For this review, use the dimensioned drawing (mm, ordinates from the lowest corner) and the shaded views. Coordinates: 2 decimals unless noted, no trailing zeros. Loops run counter-clockwise (first coordinate to the right, second up) from the corner with the lowest first, then second, coordinate; pieces in that order, holes last. Notation, with made-up numbers: (58.25, 52.25) - (80.25, 52.25) arc R13 cw to (80.25, 73.25) - close; hole circle Ø8 at (46.25, -36.5). An arc over 180 degrees is marked (long way). Use a Markdown table: item, result. Add a question column.
1) Add section A-A, the plane y = 15. Give the boundary of the cut face in (x, z).
2) Add section B-B, the plane x = 30. Give the boundary of the cut face in (y, z), and give its area (3 significant figures).
3) Clearance check with flat-ended pins moving along their axes: pin 1 (1.5 mm diameter, centred on y = 25.5, z = 3, fed in from +X); pin 2 (4 mm diameter, centred on x = 31, y = 15.5, fed in from -Z); pin 3 (1 mm diameter, centred on x = 22.5, z = 7.5, fed in from +Y); pin 4 (5 mm diameter, centred on x = 29.5, z = 3, fed in from +Y). State where each tip first meets the part, or that it passes through.
4) The part is to be moulded in two halves that separate along Y. For the marked faces 1, 2 and 3, say which applies: pulls with the +Y half, pulls with the -Y half, needs draft (parallel to the pull), parting line crosses it, or undercut.
5) To check wall thickness, follow L1, parallel to Z at x = 57, y = 24; L2, parallel to Y at x = 30, z = 7; L3, parallel to X at y = 3.75, z = 12.25 (1 decimal). State the ranges of each line that lie inside material, in increasing order. Write a range as [from, to].
6) Add section D-D, the plane z = 11.25. Give the boundary of the cut face in (x, y), and give its area (3 significant figures).
7) Add section C-C, the plane z = 4. Give the boundary of the cut face in (x, y).
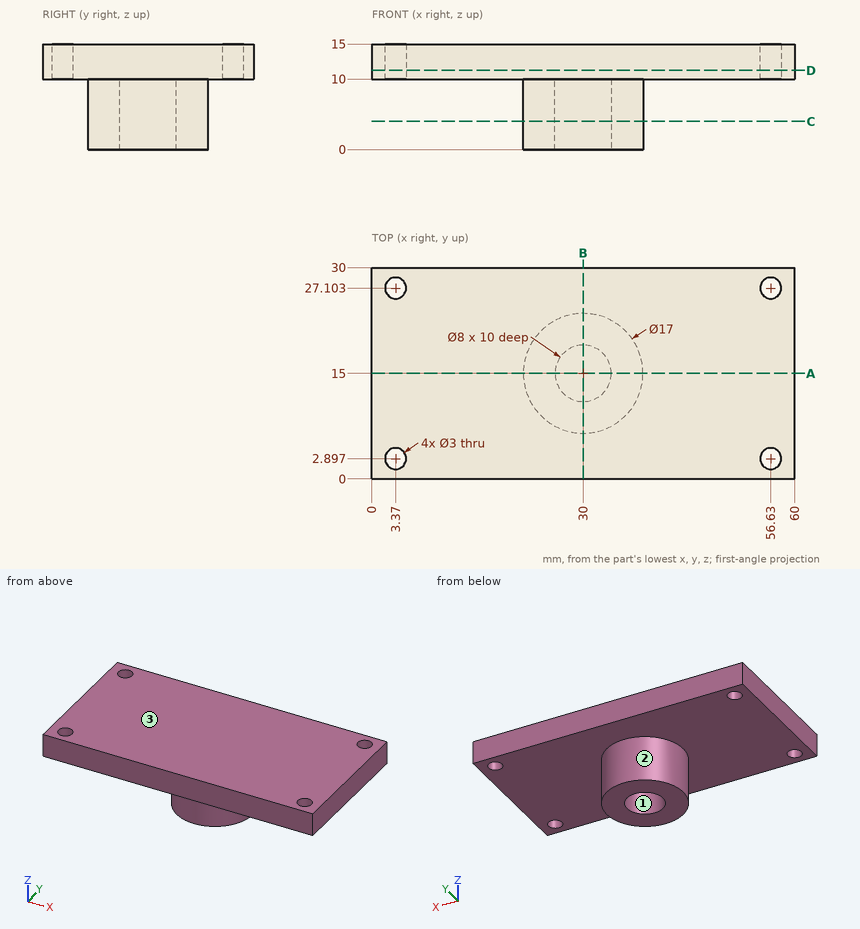
From the geometry:
| question | item | result |
|---|---|---|
| 1 | outline | (0, 10) - (21.5, 10) - (21.5, 0) - (26, 0) - (26, 10) - (34, 10) - (34, 0) - (38.5, 0) - (38.5, 10) - (60, 10) - (60, 15) - (0, 15) - close |
| 2 | outline | (0, 10) - (6.5, 10) - (6.5, 0) - (11, 0) - (11, 10) - (19, 10) - (19, 0) - (23.5, 0) - (23.5, 10) - (30, 10) - (30, 15) - (0, 15) - close |
| 2 | area | 240 mm^2 |
| 3 | pin 1 | passes through |
| 3 | pin 2 | stops at z = 10 |
| 3 | pin 3 | stops at y = 19.82 |
| 3 | pin 4 | stops at y = 23.5 |
| 4 | face 1 | undercut |
| 4 | face 2 | parting line crosses it |
| 4 | face 3 | needs draft |
| 5 | L1 | z = [10, 15] |
| 5 | L2 | y = [6.5, 11], [19, 23.5] |
| 5 | L3 | x = [0, 2.1], [4.6, 55.4], [57.9, 60] |
| 6 | outline | (0, 0) - (60, 0) - (60, 30) - (0, 30) - close; hole circle Ø3 at (3.37, 2.9); hole circle Ø3 at (3.37, 27.1); hole circle Ø3 at (56.63, 2.9); hole circle Ø3 at (56.63, 27.1) |
| 6 | area | 1,770 mm^2 |
| 7 | outline | circle Ø17 at (30, 15); hole circle Ø8 at (30, 15) |
